Answer from the drawing. Dimensions are ordinates in mm from the lowest x, y and z of the part. A direction names the side the tool comes from. Give positions to 0.01 mm unless a question says otherwise; leave off trailing zeros. Write each loop counter-clockwise with the first axis right and the second up, starting at its lowest first coordinate (ties: lowest second). Pieces come first, ordered by that corner, then holes. Notation, with made-up numbers: (75.5, 81) -> (115.5, 81) arc R16 cw to (115.5, 103) -> close; hole circle Ø8 at (-22, 37). An arc over 180 degrees is marked (long way). Put each result on its own line as item: value. Start each with the question number.
1) Find the intervals of material crossed by line 1 along X through (y, z) = (7.75, 3.8) (1 decimal); line 2 along Y through (x, z) = (8, 3.2); line 3 along X through (y, z) = (14.5, 0.6) (1 decimal), in increasing order. Write a range as from..to.
2) A cutting plane is placed at C-C (x = 7). Write down the section's boundary in (y, z).
3) For a pull along X with two mould halves and no side action, classify the marked faces 1, 2, 3 and 4 as released by +X, released by -X, zero draft, split by the parting line, or undercut.
4) For the marked faces 5 and 6, determine the directions among +Z, -Z, +X, -X, +Y, -Y from which every point of the face is accessible in a straight line to the end or side of a thin tool.
5) A cutting plane is placed at B-B (y = 9.5). Write down the section's boundary in (x, z) (1 decimal), then the cut area to 3 significant figures.
6) A cutting plane is placed at A-A (z = 4.95). Give the number of separate pieces and of enclosed holes in the cut face.
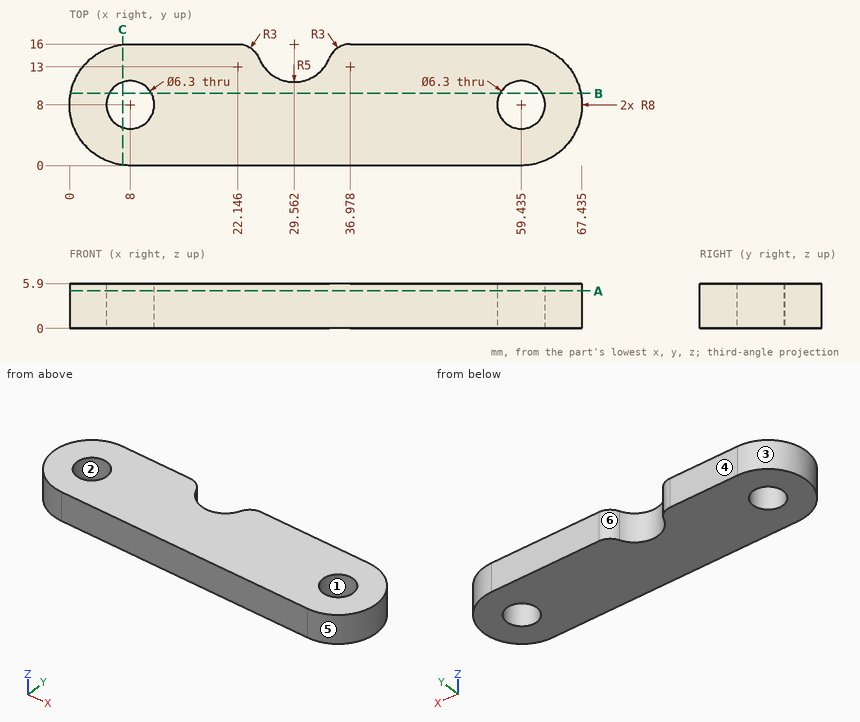
Reply:
1. line 1: x = 0..4.9, 11.1..56.3, 62.6..67.4
1. line 2: y = 0..4.85, 11.15..16
1. line 3: x = 3.3..24.7, 34.4..64.1
2. outline: (0.06, 0) -> (5.01, 0) -> (5.01, 5.9) -> (0.06, 5.9) -> close; (10.99, 0) -> (15.94, 0) -> (15.94, 5.9) -> (10.99, 5.9) -> close
3. face 1: undercut
3. face 2: undercut
3. face 3: released by -X
3. face 4: zero draft
4. face 5: +Z, -Z, +X
4. face 6: +Z, -Z, +Y
5. outline: (0.1, 0) -> (5.2, 0) -> (5.2, 5.9) -> (0.1, 5.9) -> close; (10.8, 0) -> (56.7, 0) -> (56.7, 5.9) -> (10.8, 5.9) -> close; (62.2, 0) -> (67.3, 0) -> (67.3, 5.9) -> (62.2, 5.9) -> close
5. area: 331 mm2
6. separate pieces: 1
6. enclosed holes: 2
